from build123d import *

# Parameters (mm, degrees)
F0_W          = 180
F0_H          = 105
F1_DEPTH      = 50
F2_W          = 180
F2_H          = 91
F3_DEPTH      = 1
F3_DEPTH_BACK = 43
F4_R          = 4
F5_DEPTH      = 50.001
F6_W          = 180
F6_H          = 7
F7_DEPTH      = 7
F8_R          = 1.7
F9_DEPTH      = 7


with BuildPart() as f1:
    # F0 (on Top) → F1 (new body)
    with BuildSketch(Plane.XY):
        Rectangle(F0_W, F0_H)
    extrude(amount=F1_DEPTH)

    # F2 (on face) → F3 (cut, two sides)
    with BuildSketch(Plane.XY) as f3_sk:
        Rectangle(F2_W, F2_H)
    extrude(amount=-F3_DEPTH, mode=Mode.SUBTRACT)
    extrude(f3_sk.sketch, amount=F3_DEPTH_BACK, mode=Mode.SUBTRACT)

    # F4 (on face) → F5 (cut, through all)
    with BuildSketch(Plane.XY.offset(50)):
        with Locations((0, 7.5)):
            Circle(F4_R)
    extrude(amount=-F5_DEPTH, mode=Mode.SUBTRACT)

    # F6 (on face) → F7 (join)
    with BuildSketch(Plane.XY.offset(50)):
        with Locations((0, -49)):
            Rectangle(F6_W, F6_H)
    extrude(amount=F7_DEPTH)

    # F8 (on face) → F9 (cut, through all)
    with BuildSketch(Plane(origin=(0, 52.5, 0), x_dir=(-1, 0, 0), z_dir=(0, 1, 0))):
        with Locations((-68.3, 36.3)):
            Circle(F8_R)
        with Locations((-67.4438270785, 12.9156683241)):
            Circle(F8_R)
        with Locations((-44.9, 36.3)):
            Circle(F8_R)
        with Locations((-44.0438270785, 12.9156683241)):
            Circle(F8_R)
        with Locations((44.9, 36.3)):
            Circle(F8_R)
        with Locations((45.7561729215, 12.9156683241)):
            Circle(F8_R)
        with Locations((68.3, 36.3)):
            Circle(F8_R)
        with Locations((69.1561729215, 12.9156683241)):
            Circle(F8_R)
    extrude(amount=-F9_DEPTH, mode=Mode.SUBTRACT)


solid = f1.part
Build history of the part. All positions in model axes, mm. A direction names the side the tool comes from. Coordinates: 2 decimals unless noted, no trailing zeros. Order: outer loops, then holes, each group sorted by start corner. A loop starts at its lowest first (then second) coordinate and runs counter-clockwise, first axis right, second up. Notation, with made-up numbers: (15, -28) - (30, -28) arc R8 ccw to (30, -23) - close; hole circle Ø9 at (83.25, 25). An arc over 180 degrees is marked (long way). Write each question's results on one line, items separated by ' | '. Start each with the question number.
Item 1: Band-saw the part on B-B on y = 7.5. Write the cut outline in (x, z).
Item 2: Mould opens along Y. For faces 1 (the face through (-1, 52.5, 25)), 2 (the face through (69.142, 49.049, 12.99)), 3 (the face through (-0.867, 3.595, 46.549)) say: released by +Y, released by -Y, zero draft, split by the parting line, or undercut.
Item 3: Band-saw the part on A-A on x = 0. Write the cut outline in (y, z).
Item 4: Flat gauge pins, fed straight in: pin 1 (6 mm diameter, centred on x = 53, y = -14.5, fed in from -Z); pin 2 (9 mm diameter, centred on x = 0, y = 7.5, fed in from +Z); pin 3 (3.5 mm diameter, centred on x = -22.5, z = 52, fed in from +Y). Where does each tip first touch, or does it go through?
Item 5: Wall check: probe 1 along Y at (x, z) = (0, 45.5); probe 2 along Y at (x, z) = (40, 39); probe 3 along Z at (x, y) = (44.9, 50.25). Give the ranges that are in metal, low to high. Write a range as [from, to].
Item 6: Band-saw the part on D-D on x = -61. Write the cut outline in (y, z), and give its area (3 significant figures).
Item 7: Tool access for faces 4 (the face through (-46.47, 49.05, 35.65)), 5 (the face through (-1, -52.5, 28)), 6 (the face through (-1, -45.5, 53)), 7 (the face through (-1, -45.5, 21)): list every direction of +Z, -Z, +X, -X, +Y, -Y with a clear straight run to the whole face (end or side of a thin tool).
Item 8: Band-saw the part on C-C on z = 21. Write the cut outline in (x, y), and give its area (3 significant figures).
Numbers:
1) outline: (-90, 43) - (-4, 43) - (-4, 50) - (-90, 50) - close; (4, 43) - (90, 43) - (90, 50) - (4, 50) - close
2) face 1: released by +Y | face 2: zero draft | face 3: undercut
3) outline: (-52.5, 0) - (-45.5, 0) - (-45.5, 43) - (3.5, 43) - (3.5, 50) - (-45.5, 50) - (-45.5, 57) - (-52.5, 57) - close; (11.5, 43) - (45.5, 43) - (45.5, 0) - (52.5, 0) - (52.5, 50) - (11.5, 50) - close
4) pin 1: z = 43 | pin 2: z = 50 | pin 3: y = -45.5
5) probe 1: [-52.5, 3.5], [11.5, 52.5] | probe 2: [-52.5, -45.5], [45.5, 52.5] | probe 3: [0, 11.45], [14.38, 34.6], [38, 50]
6) outline: (-52.5, 0) - (-45.5, 0) - (-45.5, 43) - (45.5, 43) - (45.5, 0) - (52.5, 0) - (52.5, 50) - (-45.5, 50) - (-45.5, 57) - (-52.5, 57) - close | area: 1,390 mm^2
7) face 4: +Y | face 5: +Z, -Z, +X, -X, -Y | face 6: +Z, +X, -X, +Y | face 7: -Z, +X, -X
8) outline: (-90, -52.5) - (90, -52.5) - (90, -45.5) - (-90, -45.5) - close; (-90, 45.5) - (90, 45.5) - (90, 52.5) - (-90, 52.5) - close | area: 2,520 mm^2
